Check sheet for the drawn part. Datum: minimum x, y, z corner. Units: mm. A direction names the side the tool comes from. Give positions to 0.01 mm unless a question says otherwise; leave off trailing zeros. Order: outer loops, then holes, each group sorted by start corner. A loop starts at its lowest first (then second) coordinate and runs counter-clockwise, first axis right, second up. Notation, with made-up numbers: (48, 79) -> (72, 79) arc R11 cw to (72, 97) -> close; hole circle Ø2 at (-32, 27). An arc over 180 degrees is marked (long way). Answer in a Markdown table with one row per item. Add a question column.
(1) Cross-section at D-D (x = 21). Record the cut outline in (y, z), then the cut area to 3 significant figures.
(2) Release check for a two-part mould opening along X. For the marked faces 1, 2 and 3 record: released by +X, released by -X, zero draft, split by the parting line, or undercut.
(3) Thickness scan on L1, parallel to Y at x = 21.5, z = 4.5; L2, parallel to Z at x = 20.25, y = 10; L3, parallel to Y at x = 10, z = 2.5. Record the ranges inside material, lowest first. Write a range as [from, to].
(4) Cross-section at B-B (y = 10). Record the cut outline in (x, z).
(5) Set-up check for the marked faces 4 and 5: record each of +Z, -Z, +X, -X, +Y, -Y from which the full face is reachable in a straight line by a thin tool's end or side.
(6) Cross-section at A-A (x = 11). Record the cut outline in (y, z).
(7) Cross-section at C-C (z = 4.5). Record the cut outline in (x, y), then the cut area to 3 significant figures.
(8) Go/stop test with flat-tipped pins: pin 1 (10 mm diameter, centred on x = 7, y = 10, fed in from -Z); pin 2 (2 mm diameter, centred on y = 16.5, z = 4, fed in from +X); pin 3 (3 mm diameter, centred on x = 21.5, z = 2.5, fed in from -Y); pin 4 (2 mm diameter, centred on y = 4.5, z = 7, fed in from -X). Record where each tip stops, or that it passes through.
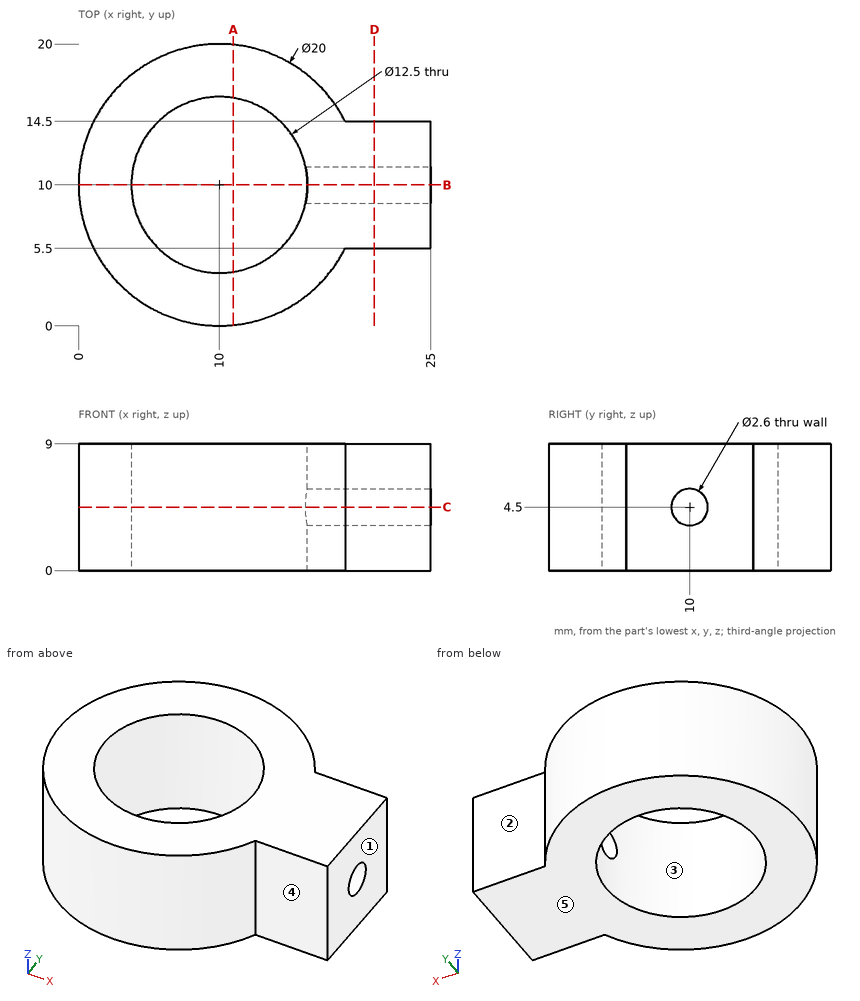
Answer below:
| question | item | result |
|---|---|---|
| 1 | outline | (5.5, 0) -> (14.5, 0) -> (14.5, 9) -> (5.5, 9) -> close; hole circle Ø2.6 at (10, 4.5) |
| 1 | area | 75.7 mm² |
| 2 | face 1 | released by +X |
| 2 | face 2 | zero draft |
| 2 | face 3 | undercut |
| 3 | L1 | y = [5.5, 8.7], [11.3, 14.5] |
| 3 | L2 | z = [0, 3.2], [5.8, 9] |
| 3 | L3 | y = [0, 3.75], [16.25, 20] |
| 4 | outline | (0, 0) -> (3.75, 0) -> (3.75, 9) -> (0, 9) -> close; (16.25, 0) -> (25, 0) -> (25, 3.2) -> (16.25, 3.2) -> close; (16.25, 5.8) -> (25, 5.8) -> (25, 9) -> (16.25, 9) -> close |
| 5 | face 4 | +Z, -Z, +X, -Y |
| 5 | face 5 | -Z, +X, -X, +Y, -Y |
| 6 | outline | (0.05, 0) -> (3.83, 0) -> (3.83, 9) -> (0.05, 9) -> close; (16.17, 0) -> (19.95, 0) -> (19.95, 9) -> (16.17, 9) -> close |
| 7 | outline | (16.11, 8.7) arc R6.25 cw (long way) to (16.11, 11.3) -> (25, 11.3) -> (25, 14.5) -> (18.93, 14.5) arc R10 ccw (long way) to (18.93, 5.5) -> (25, 5.5) -> (25, 8.7) -> close |
| 7 | area | 217 mm² |
| 8 | pin 1 | stops at z = 0 |
| 8 | pin 2 | stops at x = 18.35 |
| 8 | pin 3 | stops at y = 5.5 |
| 8 | pin 4 | stops at x = 1.07 |
